```python
from build123d import *

# Parameters (mm, degrees)
F3_DEPTH = 12.7
F1_R     = 1.5875
F4_DEPTH = 39.37
F5_DEPTH = 8.382
F6_R     = 5.08


with BuildPart() as f3:
    # F0 (on Front) → F3 (new body, symmetric)
    with BuildSketch(Plane.XZ):
        Polygon((0, 25.4), (0, 0), (2.54, 0), (2.54, 22.86), (25.4, 22.86), (25.4, 25.4), align=None)
    extrude(amount=F3_DEPTH, both=True)

    # F1 (on Top) → F4 (cut)
    with BuildSketch(Plane.XY):
        with Locations((19.05, 6.35)):
            Circle(F1_R)
        with Locations((19.05, -6.35)):
            Circle(F1_R)
    extrude(amount=F4_DEPTH, mode=Mode.SUBTRACT)

    # F2 (on Right) → F5 (cut)
    with BuildSketch(Plane.YZ):
        with BuildLine():
            ThreePointArc((7.9375, 6.35), (5.227468, 7.472532), (6.35, 4.7625))
            ThreePointArc((6.35, 4.7625), (7.472532, 5.227468), (7.9375, 6.35))
        make_face()
        with BuildLine():
            ThreePointArc((-4.7625, 6.35), (-7.472532, 7.472532), (-6.35, 4.7625))
            ThreePointArc((-6.35, 4.7625), (-5.227468, 5.227468), (-4.7625, 6.35))
        make_face()
    extrude(amount=F5_DEPTH, mode=Mode.SUBTRACT)

    # F6
    f6_edges = [f3.edges().sort_by_distance(p)[0] for p in [
        (25.4, -12.7, 24.13),
        (25.4, 12.7, 24.13),
        (1.27, -12.7, 0),
        (1.27, 12.7, 0),
    ]]
    fillet(f6_edges, radius=F6_R)


solid = f3.part
```
Source: CAD feature listing. Evaluate the final solid. Frame: model axes, mm. A direction names the side the tool comes from. Give positions to 0.01 mm unless a question says otherwise; leave off trailing zeros. Loops run counter-clockwise (first coordinate to the right, second up) from the corner with the lowest first, then second, coordinate; pieces in that order, holes last. Notation, with made-up numbers: (24, -13.5) -> (67, -13.5) arc R11 ccw to (67, 4.5) -> close; hole circle Ø5 at (-23.5, 81.25). An arc over 180 degrees is marked (long way). Use a Markdown table: item, result. Add a question column.
(1) Section query D-D (x = 12). Output: boundary loops of the cut face in (y, z), then the cut area to 3 significant figures.
(2) Ray query, line 1 (Y direction, x = 0.8, z = 6.35); line 2 (X direction, y = 6.35, z = 24.6); line 3 (Z direction, x = 0.7, y = -6.35). Return the intervals inside material, ascending.
(3) Section query B-B (y = 1.5). Output: boundary loops of the cut face in (x, z).
(4) First-contact query: pin 1 Ø7 at (y, z) = (5.5, 13.5) entering from +X; pin 2 Ø11.5 at (x, y) = (10.5, -0.5) entering from -Z. Flat tips, straight axial feed; report the tip coordinate or a pass-through.
(5) Section query C-C (z = 18.25). Output: boundary loops of the cut face in (x, y).
(6) Pull-direction query (X, two-part tool) for faces 3 (the face through (23.872, 11.251, 24.148)), 4 (the face through (17.464, -6.28, 24.112)), 5 (the face through (2, -12.7, 20)); classes: +X half, -X half, draft (parallel to the pull), parting line (faces both ways), or undercut.
(7) Section query A-A (x = 19.05). Output: boundary loops of the cut face in (y, z), then the cut area to 3 significant figures.
(8) Access query for faces 1 (the face through (2.54, 0, 11)), 2 (the face through (1, 0, 0)). Directions: +Z, -Z, +X, -X, +Y, -Y. A direction counts if a zero-diameter tool reaches every point of the face in a straight line with its end or side. Return the directions, or none.
Checked values:
| question | item | result |
|---|---|---|
| 1 | outline | (-12.7, 22.86) -> (12.7, 22.86) -> (12.7, 25.4) -> (-12.7, 25.4) -> close |
| 1 | area | 64.5 mm^2 |
| 2 | line 1 | -12.7 to -7.94, -4.76 to 4.76, 7.94 to 12.7 |
| 2 | line 2 | 0 to 17.46, 20.64 to 25.4 |
| 2 | line 3 | 0 to 4.76, 7.94 to 25.4 |
| 3 | outline | (0, 0) -> (2.54, 0) -> (2.54, 22.86) -> (25.4, 22.86) -> (25.4, 25.4) -> (0, 25.4) -> close |
| 4 | pin 1 | x = 2.54 |
| 4 | pin 2 | z = 22.86 |
| 5 | outline | (0, -12.7) -> (2.54, -12.7) -> (2.54, 12.7) -> (0, 12.7) -> close |
| 6 | face 3 | +X half |
| 6 | face 4 | undercut |
| 6 | face 5 | draft |
| 7 | outline | (-12.7, 22.86) -> (-7.94, 22.86) -> (-7.94, 25.4) -> (-12.7, 25.4) -> close; (-4.76, 22.86) -> (4.76, 22.86) -> (4.76, 25.4) -> (-4.76, 25.4) -> close; (7.94, 22.86) -> (12.7, 22.86) -> (12.7, 25.4) -> (7.94, 25.4) -> close |
| 7 | area | 48.4 mm^2 |
| 8 | face 1 | -Z, +X, +Y, -Y |
| 8 | face 2 | -Z, +X, -X, +Y, -Y |
